```python
from build123d import *

# Parameters (mm, degrees)
BOSS_EXTRUDE1_START     = -9
BOSS_EXTRUDE1_OUTLINE_R = 1
BOSS_EXTRUDE1_DEPTH     = 9
BOSS_EXTRUDE1_START_2   = -10
BOSS_EXTRUDE1_2_DEPTH   = 1
BOSS_EXTRUDE2_START     = -40
BOSS_EXTRUDE2_DEPTH     = 40
CUT_EXTRUDE6_DEPTH      = 31
BOSS_EXTRUDE5_DEPTH     = 10
CHAMFER5_SIZE           = 10
SKETCH17_R              = 1.5000000000000002
SKETCH17_R_2            = 1.5000000000000004
SKETCH17_R_3            = 1.5
CUT_EXTRUDE7_DEPTH      = 81.58306320285853


with BuildPart() as part:
    # Boss-Extrude1: read off the stored shape, not the designer's step
    # Boss-Extrude1 outline → Boss-Extrude1 (new body)
    with BuildSketch(Plane(origin=(4.6139639648499715, 0, 0), x_dir=(0, 0, -1), z_dir=(1, 0, 0)).offset(BOSS_EXTRUDE1_START)):
        with BuildLine():
            ThreePointArc((-10.591117285, -4.446613705), (-10.456680456, -4.73552608), (-10.314619658, -5.020766944))
            ThreePointArc((-10.314619658, -5.020766944), (-8.502494616, -5.018593908), (-6.859954563, -4.253176333))
            ThreePointArc((-6.859954563, -4.253176333), (-6.387568746, -4.905897262), (-5.856328627, -5.51168345))
            ThreePointArc((-5.856328627, -5.51168345), (-6.968055133, -6.942720161), (-7.373409443, -8.708927899))
            ThreePointArc((-7.373409443, -8.708927899), (-7.126931664, -8.910899), (-6.875177934, -9.106254268))
            ThreePointArc((-6.875177934, -9.106254268), (-5.243452532, -8.318044841), (-4.095677319, -6.915756016))
            ThreePointArc((-4.095677319, -6.915756016), (-3.386867407, -7.298876727), (-2.645395822, -7.614174775))
            ThreePointArc((-2.645395822, -7.614174775), (-3.026123234, -9.385854353), (-2.625006031, -11.153029182))
            ThreePointArc((-2.625006031, -11.153029182), (-2.315305249, -11.228056157), (-2.003721502, -11.294833322))
            ThreePointArc((-2.003721502, -11.294833322), (-0.875578967, -9.876702048), (-0.449899552, -8.115282471))
            ThreePointArc((-0.449899552, -8.115282471), (0.354945958, -8.15292121), (1.159791469, -8.115282471))
            ThreePointArc((1.159791469, -8.115282471), (1.585470883, -9.876702048), (2.713613419, -11.294833322))
            ThreePointArc((2.713613419, -11.294833322), (3.025197166, -11.228056157), (3.334897948, -11.153029182))
            ThreePointArc((3.334897948, -11.153029182), (3.736015151, -9.385854353), (3.355287739, -7.614174775))
            ThreePointArc((3.355287739, -7.614174775), (4.096759324, -7.298876727), (4.805569236, -6.915756016))
            ThreePointArc((4.805569236, -6.915756016), (5.953344449, -8.318044841), (7.585069851, -9.106254268))
            ThreePointArc((7.585069851, -9.106254268), (7.836823581, -8.910899), (8.083301359, -8.708927899))
            ThreePointArc((8.083301359, -8.708927899), (7.677947049, -6.942720161), (6.566220544, -5.51168345))
            ThreePointArc((6.566220544, -5.51168345), (7.097460663, -4.905897262), (7.56984648, -4.253176333))
            ThreePointArc((7.56984648, -4.253176333), (9.212386533, -5.018593908), (11.024511575, -5.020766944))
            ThreePointArc((11.024511575, -5.020766944), (11.166572373, -4.73552608), (11.301009202, -4.446613705))
            ThreePointArc((11.301009202, -4.446613705), (10.169468771, -3.031192163), (8.546934241, -2.224232691))
            ThreePointArc((8.546934241, -2.224232691), (8.762724273, -1.447941745), (8.90512419, -0.654899984))
            ThreePointArc((8.90512419, -0.654899984), (10.717103882, -0.631845971), (12.350714974, 0.152447781))
            ThreePointArc((12.350714974, 0.152447781), (12.354945958, 0.47107879), (12.350714974, 0.789709799))
            ThreePointArc((12.350714974, 0.789709799), (10.717103881, 1.57400355), (8.90512419, 1.597057563))
            ThreePointArc((8.90512419, 1.597057563), (8.762724273, 2.390099324), (8.546934241, 3.16639027))
            ThreePointArc((8.546934241, 3.16639027), (10.169468771, 3.973349742), (11.301009202, 5.388771284))
            ThreePointArc((11.301009202, 5.388771284), (11.166572373, 5.677683659), (11.024511575, 5.962924523))
            ThreePointArc((11.024511575, 5.962924523), (9.212386533, 5.960751487), (7.56984648, 5.195333912))
            ThreePointArc((7.56984648, 5.195333912), (7.255600261, 5.643539152), (6.913552392, 6.070905362))
            Line((6.913552392, 6.070905362), (7.795891782, 6.27229357))
            Line((7.795891782, 6.27229357), (13.400397117, 33.194406922))
            Line((13.400397117, 33.194406922), (5.612164429, 67.316883848))
            Line((5.612164429, 67.316883848), (-16.111603154, 72.615744291))
            Line((-16.111603154, 72.615744291), (-13.886393815, 62.866465169))
            ThreePointArc((-13.886393815, 62.866465169), (-0.835936603, 47.895101758), (-6.098161126, 28.743988243))
            Line((-6.098161126, 28.743988243), (-2.315305249, 12.170213736))
            ThreePointArc((-2.315305249, 12.170213736), (-2.470404693, 12.133728304), (-2.625006031, 12.095186762))
            ThreePointArc((-2.625006031, 12.095186762), (-3.026123234, 10.328011932), (-2.645395822, 8.556332354))
            ThreePointArc((-2.645395822, 8.556332354), (-3.386867407, 8.241034306), (-4.095677319, 7.857913595))
            ThreePointArc((-4.095677319, 7.857913595), (-5.243452532, 9.260202421), (-6.875177934, 10.048411847))
            ThreePointArc((-6.875177934, 10.048411847), (-7.126931664, 9.853056579), (-7.373409443, 9.651085478))
            ThreePointArc((-7.373409443, 9.651085478), (-6.968055133, 7.88487774), (-5.856328627, 6.45384103))
            ThreePointArc((-5.856328627, 6.45384103), (-6.387568746, 5.848054841), (-6.859954563, 5.195333912))
            ThreePointArc((-6.859954563, 5.195333912), (-8.502494616, 5.960751487), (-10.314619658, 5.962924523))
            ThreePointArc((-10.314619658, 5.962924523), (-10.456680456, 5.677683659), (-10.591117285, 5.388771284))
            ThreePointArc((-10.591117285, 5.388771284), (-9.459576854, 3.973349742), (-7.837042324, 3.16639027))
            ThreePointArc((-7.837042324, 3.16639027), (-8.052832356, 2.390099324), (-8.195232274, 1.597057563))
            ThreePointArc((-8.195232274, 1.597057563), (-10.007211965, 1.57400355), (-11.640823057, 0.789709799))
            ThreePointArc((-11.640823057, 0.789709799), (-11.645054042, 0.47107879), (-11.640823057, 0.152447781))
            ThreePointArc((-11.640823057, 0.152447781), (-10.007211965, -0.631845971), (-8.195232274, -0.654899984))
            ThreePointArc((-8.195232274, -0.654899984), (-8.052832356, -1.447941745), (-7.837042324, -2.224232691))
            ThreePointArc((-7.837042324, -2.224232691), (-9.459576854, -3.031192163), (-10.591117285, -4.446613705))
        make_face()
        with Locations((0.354945958, 0.47107879)):
            Circle(BOSS_EXTRUDE1_OUTLINE_R, mode=Mode.SUBTRACT)
    extrude(amount=BOSS_EXTRUDE1_DEPTH)

    # Boss-Extrude1 2 outline → Boss-Extrude1 2 (add)
    with BuildSketch(Plane(origin=(4.6139639648499715, 0, 0), x_dir=(0, 0, -1), z_dir=(1, 0, 0)).offset(BOSS_EXTRUDE1_START_2)):
        with BuildLine():
            Line((-6.098161126, 28.743988243), (-0.535137777, 4.370790438))
            Line((-0.535137777, 4.370790438), (7.795891782, 6.27229357))
            Line((7.795891782, 6.27229357), (13.400397117, 33.194406922))
            Line((13.400397117, 33.194406922), (5.612164429, 67.316883848))
            Line((5.612164429, 67.316883848), (-16.111603154, 72.615744291))
            Line((-16.111603154, 72.615744291), (-13.886393815, 62.866465169))
            ThreePointArc((-13.886393815, 62.866465169), (-0.835936603, 47.895101758), (-6.098161126, 28.743988243))
        make_face()
    extrude(amount=BOSS_EXTRUDE1_2_DEPTH)

    # Sketch2 → Boss-Extrude2 (add)
    with BuildSketch(Plane(origin=(4.6139639648499715, 0, 0), x_dir=(0, 0, -1), z_dir=(1, 0, 0)).offset(BOSS_EXTRUDE2_START)):
        with BuildLine():
            Line((-16.11160315441779, 72.61574429110016), (5.612164428781802, 67.31688384840837))
            Line((5.612164428781802, 67.31688384840837), (13.400397117252913, 33.19440692204444))
            Line((13.400397117252913, 33.19440692204444), (8.3052597658331, 8.719121931463299))
            Line((8.3052597658331, 8.719121931463299), (-1.647742447257206, 9.245429999281619))
            Line((-1.647742447257206, 9.245429999281619), (-6.098161126383539, 28.743988242918082))
            ThreePointArc((-6.098161126383539, 28.743988242918082), (-0.8359366030316124, 47.895101758418704), (-13.886393814854628, 62.866465169281916))
            Line((-13.886393814854628, 62.866465169281916), (-16.11160315441779, 72.61574429110016))
        make_face()
    extrude(amount=BOSS_EXTRUDE2_DEPTH)

    # Sketch13 → Cut-Extrude6 (cut)
    with BuildSketch(Plane.ZY.offset(35.386036035150035)):
        Polygon((-7.7958917817334035, 6.272293570213381), (-10.852828441543005, 20.95676442675387), (5.0777102899861175, 24.273101006715667), (0.5351377774756237, 4.370790438372502), align=None)
    extrude(amount=-CUT_EXTRUDE6_DEPTH, mode=Mode.SUBTRACT)

    # Sketch15 → Boss-Extrude5 (add)
    with BuildSketch(Plane.ZY.offset(4.3860360351500285)):
        Polygon((-10.852828441543005, 20.95676442675387), (5.077710289986116, 24.273101006715674), (2.315305249124831, 12.17021373582128), (-9.187430109019209, 12.956764426753871), align=None)
    extrude(amount=BOSS_EXTRUDE5_DEPTH)

    # Chamfer5
    chamfer5_edges = [part.edges().sort_by_distance(p)[0] for p in [
        (-14.386036035150028, 12.563489081287575, -3.436062429947189),
    ]]
    chamfer(chamfer5_edges, length=CHAMFER5_SIZE - 0.0001)  # a hair under: the kernel refuses the full size

    # Sketch17 → Cut-Extrude7 (cut, through all)
    with BuildSketch(Plane.ZY.offset(4.3860360351500285)):
        with Locations((-0.35494595834961384, 7.471078789645248)):
            Circle(SKETCH17_R)
        with Locations((6.645054041650483, 0.47107878964532196)):
            Circle(SKETCH17_R)
        with Locations((-0.354945958349467, -6.528921210354753)):
            Circle(SKETCH17_R_2)
        with Locations((-7.354945958349516, 0.4710787896452233)):
            Circle(SKETCH17_R_3)
    extrude(amount=-CUT_EXTRUDE7_DEPTH, mode=Mode.SUBTRACT)


solid = part.part
```
The listing builds one solid part. Answer for the finished solid, in the listing's coordinates (mm). Give positions to 0.01 mm unless a question says otherwise; leave off trailing zeros. Loops run counter-clockwise (first coordinate to the right, second up) from the corner with the lowest first, then second, coordinate; pieces in that order, holes last. Notation, with made-up numbers: M -31.75,12 L 18.25,12 A20 cw 18.25,23 Z; hole C -9,29 d9. An arc over 180 degrees is marked long. One line per item, written item: value.
1. Find the intervals of material crossed by probe 1 along Z at (x, y) = (0, 0); probe 2 along X at (y, z) = (-3.5, -4.25); probe 3 along Y at (x, z) = (-16, 3.25), in increasing order.
Found:
probe 1: -12.14 to -8.78, -5.93 to -1.24, 0.53 to 5.22, 8.07 to 11.43
probe 2: -4.39 to 4.61
probe 3: 23.89 to 32.51, 53.94 to 69.48
2. Section C-C on y = 31 is taken. Determine the outline of the cut face in (x, z).
Found:
outline: M -35.39,-12.94 L 4.61,-12.94 L 4.61,4.23 L -35.39,4.23 Z
3. Section A-A on x = -29.5 is taken. Determine the outline of the cut face in (y, z), plus the area to 3 significant figures.
Found:
outline: M 20.96,-10.85 L 33.19,-13.4 L 67.32,-5.61 L 72.62,16.11 L 62.87,13.89 A21 cw 28.74,6.1 L 24.27,5.08 Z
area: 716 mm^2
4. For a pull along Z with two mould halves and no side action, classify faces 1 (the face through (4.614, 31, -2)), 2 (the face through (0.051, -9.854, -1.574)) as pulls with the +Z half, pulls with the -Z half, needs draft (parallel to the pull), parting line crosses it, or undercut.
Found:
face 1: needs draft
face 2: undercut
5. Each of these flat-tipped pins is pushed along its axis until it touches: P1, Ø3.5, axis at y = -6.53, z = -0.35, coming from the -X side; P2, Ø2.5, axis at y = 7.47, z = -0.35, coming from the -X side; P3, Ø1.5, axis at x = 0.5, y = 15.5, coming from the -Z side; P4, Ø5, axis at x = -9.5, z = 9.5, coming from the +Y side. Where does it stop, or does it pass through?
Found:
P1: x = -4.39
P2: through
P3: z = -9.87
P4: y = 71.61
6. Section D-D on x = -11 is taken. Determine the outline of the cut face in (y, z), plus the area to 3 significant figures.
Found:
outline: M 18.7,3.81 L 19.68,-10.59 L 33.19,-13.4 L 67.32,-5.61 L 72.62,16.11 L 62.87,13.89 A21 cw 28.74,6.1 Z
area: 768 mm^2
7. Section B-B on z = -10 is taken. Determine the outline of the cut face in (x, y).
Found:
outline: M -35.39,21.13 L -12.49,21.13 L -8.22,16.86 L 4.61,16.86 L 4.61,48.09 L -35.39,48.09 Z; M -4.39,-5.12 L 4.61,-5.12 L 4.61,-2.9 L -4.39,-2.9 Z; M -4.39,-0.74 L 4.61,-0.74 L 4.61,1.68 L -4.39,1.68 Z; M -4.39,3.84 L 4.61,3.84 L 4.61,6.06 L -4.39,6.06 Z
